Here's how the part is built. I have some questions about the finished solid (model axes, mm). Face numbers are marked on the shaded views. A direction names the side the tool comes from. Coordinates: 2 decimals unless noted, no trailing zeros. Order: outer loops, then holes, each group sorted by start corner. A loop starts at its lowest first (then second) coordinate and runs counter-clockwise, first axis right, second up. Notation, with made-up numbers: (16.25, 82.25) - (22.25, 82.25) arc R7 cw to (22.25, 95.25) - close; hole circle Ø9 at (-32, 88). An arc over 180 degrees is marked (long way). Answer as CSV lines item,"result". Start each with the question number.
Item 1: I'm going to push flat-ended pins straight in: pin 1 (2 mm diameter, centred on x = -3.5, y = 4, fed in from -Z); pin 2 (10 mm diameter, centred on x = 0.5, z = 9.5, fed in from -Y); pin 3 (1.5 mm diameter, centred on x = -5.5, y = -1, fed in from +Z). Where does each tip first touch, or does it pass through?
Item 2: Imagine slicing it at D-D on x = 12.5. List the corners of the cut face in (y, z) for me, and give its area (3 significant figures).
Item 3: Imagine slicing it at B-B on z = 9.5. List the corners of the cut face in (x, y) for me (3 decimals), and give its area (3 significant figures).
Item 4: I need wall thicknesses on line 1 (X direction, y = 0.5, z = -10.16) (3 decimals); line 2 (Z direction, x = 5.5, y = 3); line 3 (Y direction, x = -10.5, z = 4.25). Which ranges of each line are inside material? Lowest first, please.
Item 5: Imagine slicing it at C-C on z = 0. List the corners of the cut face in (x, y) for me (3 decimals), and give its area (3 significant figures).
Item 6: On a 3-axis mill with a long thin cutter (end or side, diameter ignored), from which of +Z, -Z, +X, -X, +Y, -Y can I reach the whole of each face in a straight line? I mean the marked faces 1, 2, 3 and 4. Say none if no direction works.
Item 7: Imagine slicing it at A-A on y = 0.5. List the corners of the cut face in (x, z) for me (3 decimals), and give its area (3 significant figures).
from build123d import *

# Parameters (mm, degrees)
PCB_DEPTH            = 1.6
M2_CLEARANCE_HOLE1_D = 2.4
SKETCH4_W            = 15
SKETCH4_H            = 15
ANTENNA_DEPTH        = 4.4
SKETCH5_R            = 6.5
BATTERY_HOLDER_DEPTH = 3.5


with BuildPart() as part:
    # Sketch1 → PCB (new body)
    with BuildSketch(Plane(origin=(0, 0, 0), x_dir=(1, 0, 0), z_dir=(0, 1, 0))):
        with BuildLine():
            Line((-14.605, -12.7), (14.605, -12.7))
            ThreePointArc((14.605, -12.7), (16.401051224, -11.956051224), (17.145, -10.16))
            Line((17.145, -10.16), (17.145, 10.16))
            ThreePointArc((17.145, 10.16), (16.401051224, 11.956051224), (14.605, 12.7))
            Line((14.605, 12.7), (-14.605, 12.7))
            ThreePointArc((-14.605, 12.7), (-16.401051224, 11.956051224), (-17.145, 10.16))
            Line((-17.145, 10.16), (-17.145, -10.16))
            ThreePointArc((-17.145, -10.16), (-16.401051224, -11.956051224), (-14.605, -12.7))
        make_face()
    extrude(amount=PCB_DEPTH)

    # M2 Clearance Hole1 (through all)
    with Locations(Plane(origin=(0, 1.6, 0), x_dir=(1, 0, 0), z_dir=(0, 1, 0))):
        with Locations((-14.605, -10.16), (-14.605, 10.16)):
            Hole(M2_CLEARANCE_HOLE1_D / 2)

    # Sketch4 → Antenna (add)
    with BuildSketch(Plane(origin=(0, 1.6, 0), x_dir=(1, 0, 0), z_dir=(0, 1, 0))):
        with Locations((-0.045, -1.2)):
            Rectangle(SKETCH4_W, SKETCH4_H)
    extrude(amount=ANTENNA_DEPTH)

    # Sketch5 → Battery Holder (add)
    with BuildSketch(Plane.XZ):
        with Locations((-9.645, 0)):
            Circle(SKETCH5_R)
    extrude(amount=BATTERY_HOLDER_DEPTH)


solid = part.part
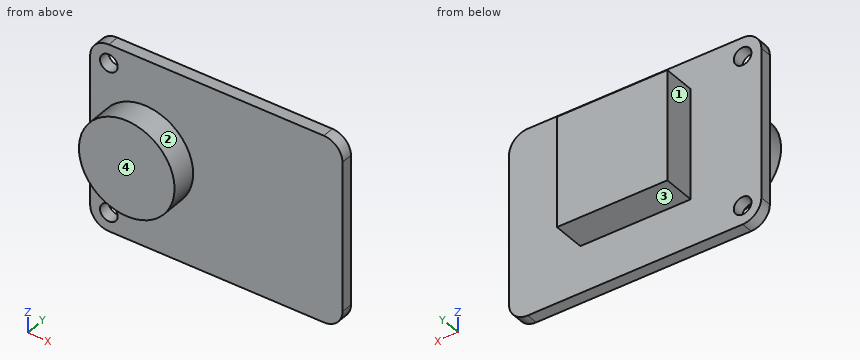
Responses:
1,pin 1,"stops at z = -6.3"
1,pin 2,"stops at y = 0"
1,pin 3,"stops at z = 5.54"
2,outline,"(0, -12.7) - (1.6, -12.7) - (1.6, 12.7) - (0, 12.7) - close"
2,area,"40.6 mm^2"
3,outline,"(-17.145, 0) - (-15.607, 0) - (-15.607, 1.6) - (-17.145, 1.6) - close; (-13.603, 0) - (17.145, 0) - (17.145, 1.6) - (-13.603, 1.6) - close"
3,area,"51.7 mm^2"
4,line 1,"x = -17.145 to -15.805, -13.405 to 17.145"
4,line 2,"z = -6.3 to 8.7"
4,line 3,"y = -3.5 to 1.6"
5,outline,"(-17.145, 0) - (-16.145, 0) - (-16.145, -3.5) - (-3.145, -3.5) - (-3.145, 0) - (17.145, 0) - (17.145, 1.6) - (7.455, 1.6) - (7.455, 6) - (-7.545, 6) - (-7.545, 1.6) - (-17.145, 1.6) - close"
5,area,"166 mm^2"
6,face 1,"+Z, -Z, -X, +Y"
6,face 2,"-Y"
6,face 3,"-Z, +X, -X, +Y"
6,face 4,"+Z, -Z, +X, -X, -Y"
7,outline,"(-17.145, -10.16) arc R2.54 ccw to (-14.605, -12.7) - (14.605, -12.7) arc R2.54 ccw to (17.145, -10.16) - (17.145, 10.16) arc R2.54 ccw to (14.605, 12.7) - (-14.605, 12.7) arc R2.54 ccw to (-17.145, 10.16) - close; hole circle Ø2.4 at (-14.605, -10.16); hole circle Ø2.4 at (-14.605, 10.16)"
7,area,"856 mm^2"
